```python
from build123d import *

# Parameters (mm, degrees)
F1_DEPTH = 50
F2_R     = 12.5
F2_R_2   = 2.5
F3_DEPTH = 7.501
F4_R     = 12.5
F4_R_2   = 2.5
F5_DEPTH = 7.501


with BuildPart() as f1:
    # F0 (on Right) → F1 (new body)
    with BuildSketch(Plane.YZ):
        Polygon((7.5, 50), (0, 50), (0, 0), (50, 0), (50, 7.5), (7.5, 7.5), align=None)
    extrude(amount=F1_DEPTH)

    # F2 (on face) → F3 (cut, through all)
    with BuildSketch(Plane(origin=(0, 7.5, 0), x_dir=(-1, 0, 0), z_dir=(0, 1, 0))):
        with Locations((-25, 28.75)):
            Circle(F2_R)
        with Locations((-42.262121, 43.422803)):
            Circle(F2_R_2)
        with Locations((-7.737879, 43.422803)):
            Circle(F2_R_2)
        with Locations((-7.737879, 14.077197)):
            Circle(F2_R_2)
        with Locations((-42.262121, 14.077197)):
            Circle(F2_R_2)
    extrude(amount=-F3_DEPTH, mode=Mode.SUBTRACT)

    # F4 (on face) → F5 (cut, through all)
    with BuildSketch(Plane.XY.offset(7.5)):
        with Locations((25, 28.75)):
            Circle(F4_R)
        with Locations((7.737879, 43.422803)):
            Circle(F4_R_2)
        with Locations((42.262121, 43.422803)):
            Circle(F4_R_2)
        with Locations((42.262121, 14.077197)):
            Circle(F4_R_2)
        with Locations((7.737879, 14.077197)):
            Circle(F4_R_2)
    extrude(amount=-F5_DEPTH, mode=Mode.SUBTRACT)


solid = f1.part
```
Geometry: final body of the model. Coordinates: model frame, mm. A direction names the side the tool comes from. Round coordinates to 2 decimals unless told otherwise and drop trailing zeros. Loops run counter-clockwise (first coordinate to the right, second up) from the corner with the lowest first, then second, coordinate; pieces in that order, holes last.
Item 1: Reachability of faces 1 (the cylindrical face through (34.92, 3.802, 21.144)), 2 (the flat face through (25, 7.5, 14)) from +Z, -Z, +X, -X, +Y, -Y: full face, straight path, thin tool, end or side. Return the list, or none.
Checked values:
face 1: +Y, -Y
face 2: +Z, +X, -X, +Y
Item 2: Line query: L1, parallel to Z at x = 46, y = 36.5; L2, parallel to X at y = 34, z = 6. Output: solid intervals per line, ascending.
Checked values:
L1: z = 0 to 7.5
L2: x = 0 to 13.66, 36.34 to 50
Item 3: Section B-B, the plane z = 28.75. Output: boundary loops of the cut face in (x, y).
Checked values:
outline: (0, 0) - (12.5, 0) - (12.5, 7.5) - (0, 7.5) - close; (37.5, 0) - (50, 0) - (50, 7.5) - (37.5, 7.5) - close
Item 4: Section A-A, the plane x = 25. Output: boundary loops of the cut face in (y, z).
Checked values:
outline: (0, 0) - (16.25, 0) - (16.25, 7.5) - (7.5, 7.5) - (7.5, 16.25) - (0, 16.25) - close; (0, 41.25) - (7.5, 41.25) - (7.5, 50) - (0, 50) - close; (41.25, 0) - (50, 0) - (50, 7.5) - (41.25, 7.5) - close
Item 5: Mould query, pull axis Z, two halves, no side actions, for faces 3 (the flat face through (25, 43, 7.5)), 4 (the flat face through (25, 0, 14)), 5 (the cylindrical face through (9.722, 3.802, 12.556)), 6 (the cylindrical face through (42.804, 3.802, 11.637)). Classes: released by +Z, released by -Z, zero draft, split by the parting line, or undercut.
Checked values:
face 3: released by +Z
face 4: zero draft
face 5: undercut
face 6: undercut
Item 6: Section D-D, the plane y = 15.5. Output: boundary loops of the cut face in (x, z), plus the area to 3 significant figures.
Checked values:
outline: (0, 0) - (5.68, 0) - (5.68, 7.5) - (0, 7.5) - close; (9.79, 0) - (40.21, 0) - (40.21, 7.5) - (9.79, 7.5) - close; (44.32, 0) - (50, 0) - (50, 7.5) - (44.32, 7.5) - close
area: 313 mm2
Item 7: Contact query for flat-ended pins moving along their axis: P1, Ø6, axis at x = 42.26, y = 14.08, coming from the +Z side; P2, Ø8, axis at x = 9.5, y = 10.5, coming from the +Z side; P3, Ø3, axis at x = 6, z = 35.5, coming from the +Y side. Output: stop coordinate, or through.
Checked values:
P1: stops at z = 7.5
P2: stops at z = 50
P3: stops at y = 7.5
